Could you check a few things on this model? Use its own coordinates, in mm. A direction names the side the tool comes from. Give positions to 0.01 mm unless a question says otherwise; leave off trailing zeros. Loops run counter-clockwise (first coordinate to the right, second up) from the corner with the lowest first, then second, coordinate; pieces in that order, holes last. Notation, with made-up numbers: (66.25, 67.5) -> (80.25, 67.5) arc R21 cw to (80.25, 88.5) -> close; hole circle Ø7 at (21.25, 58.5). An arc over 180 degrees is marked (long way). Write item = value, one per line. Start each with the question number.
1) I'm going to push flat-ended pins straight in: pin 1 Ø3 at (x, z) = (4, 94.5) entering from +Y; pin 2 Ø7.5 at (x, z) = (12, -6.5) entering from +Y; pin 3 Ø5 at (x, z) = (26.5, -4.5) entering from -Y; pin 4 Ø3 at (x, z) = (26.1, 105.5) entering from -Y. Where does each tip first touch, or does it pass through?
2) I want a section at C-C (x = 6.5). List the corners of the cut face in (y, z) for me, and give its area (3 significant figures).
3) I want a section at B-B (z = 84.5). List the corners of the cut face in (x, y) for me.
4) If we mould it in two halves opening along Z, with no side actions, what happens to faces 1 (the face through (24, 13, 50)), 2 (the face through (11, 5, -9.5)), 3 (the face through (27.484, 1.528, 102.838))? For each: +Z half, -Z half, draft (parallel to the pull), parting line (faces both ways), or undercut.
5) I want a section at A-A (y = 1.5). List the corners of the cut face in (x, z) for me, and give its area (3 significant figures).
6) On a 3-axis mill with a long thin cutter (end or side, diameter ignored), from which of +Z, -Z, +X, -X, +Y, -Y can I reach the whole of each face in a straight line? I mean faces 4 (the face through (1.55, 9, -5)), 5 (the face through (21.6, 8, 50)), 6 (the face through (-5.15, 1.53, 102.57)). Say none if no direction works.
7) I need wall thicknesses on probe 1 along Z at (x, y) = (26.1, 5.5); probe 2 along Z at (x, y) = (26, 2); probe 3 along X at (y, z) = (8.25, -4.5). Which ranges of each line are inside material? Lowest first, please. Write a range as from..to.
Autodesk Fusion 360 part; units mm, degrees
sketch "Sketch1" plane through (0, 0, 0) normal (0, 1, 0) x (1, 0, 0)
  line L0 (0, 0) -> (21.6, 0)
  line L1 (21.6, 0) -> (21.6, -101)
  line L2 (21.6, -101) -> (0, -101)
  line L3 (0, -101) -> (0, 0)
  line L4 (-9.5, 9.5) -> (31.1, 9.5)
  line L5 (31.1, 9.5) -> (31.1, -110.5)
  line L6 (31.1, -110.5) -> (-9.5, -110.5)
  line L7 (-9.5, -110.5) -> (-9.5, 9.5)
  circle A0 centre (-4.5, -105.5) radius 1.7
  circle A1 centre (26.1, -105.5) radius 1.7
  circle A2 centre (26.1, 4.5) radius 1.7
  circle A3 centre (-4.5, 4.5) radius 1.7
  circle A4 centre (-4.5, 4.5) radius 3
  circle A5 centre (26.1, 4.5) radius 3
  circle A6 centre (26.1, -105.5) radius 3
  circle A7 centre (-4.5, -105.5) radius 3
  dimension "d1" = 21.6
  dimension "d2" = 101
  dimension "d3" = 40.6
  dimension "d4" = 120
  dimension "d5" = 9.5
  dimension "d6" = 9.5
  dimension "d7" = 3.4
  dimension "d8" = 3.4
  dimension "d9" = 3.4
  dimension "d10" = 3.4
  dimension "d11" = 5
  dimension "d12" = 5
  dimension "d13" = 5
  dimension "d14" = 5
  dimension "d15" = 5
  dimension "d16" = 5
  dimension "d17" = 5
  dimension "d18" = 5
  dimension "d19" = 6
  dimension "d20" = 6
  dimension "d21" = 6
  dimension "d22" = 6
extrude "Extrude1" add sketch "Sketch1" along normal blind 9.9 from surface at 3.1 contours A4 | A5 | A6 | A7 makes body 1 at (29.0963, 9.7, -4.3505) makes body 2 at (-1.5037, 9.7, -4.3505) makes body 3 at (28.6599, 9.7, 103.9357) makes body 4 at (-7.2644, 9.7, 106.6653)
extrude "Extrude2" add sketch "Sketch1" along normal blind 13 contours L4 L5 L6 L7 bodies 1 2 3 4
extrude "Extrude3" add sketch "Sketch1" along normal blind 3 contours L0 L1 L2 L3 bodies 1
sketch "Sketch2" plane through (0, 13, 0) normal (0, 1, 0) x (-1, 0, 0)
  circle A0 centre (-26.1, -4.5) radius 1.7
  circle A1 centre (4.5, 105.5) radius 1.7
  line L0 (-21.6, 101) -> (0, 101)
  line L1 (0, 101) -> (0, 0)
  line L2 (0, 0) -> (-21.6, 0)
  line L3 (-21.6, 0) -> (-21.6, 101)
  line L4 (9.5, 110.5) -> (-31.1, 110.5)
  line L5 (-31.1, 110.5) -> (-31.1, -9.5)
  line L6 (-31.1, -9.5) -> (9.5, -9.5)
  line L7 (9.5, -9.5) -> (9.5, 110.5)
  circle A2 centre (4.5, -4.5) radius 1.7
  circle A3 centre (-26.1, 105.5) radius 1.7
  line L8 (-1.55, -9.5) -> (-20.05, -9.5)
  line L9 (-20.05, -9.5) -> (-20.05, 0)
  line L10 (-20.05, 0) -> (-1.55, 0)
  line L11 (-1.55, 0) -> (-1.55, -9.5)
  dimension "d30" = 11.05
  dimension "d31" = 18.5
extrude "Extrude4" cut sketch "Sketch2" against normal blind 7.5 contours L2 L6 L8 L9 L10 L11 bodies 1
fillet "Fillet1" radius 5 4 edges at (31.1, 6.5, -9.5) (-9.5, 6.5, -9.5) (-9.5, 6.5, 110.5) (31.1, 6.5, 110.5) on bodies 1
Answer list:
q1.pin_1 = 3
q1.pin_2 = 5.5
q1.pin_3 = 3.1
q1.pin_4 = through
q2.outline = (0, -9.5) -> (5.5, -9.5) -> (5.5, 0) -> (3, 0) -> (3, 101) -> (13, 101) -> (13, 110.5) -> (0, 110.5) -> close
q2.area = 479 mm^2
q3.outline = (-9.5, 0) -> (31.1, 0) -> (31.1, 13) -> (21.6, 13) -> (21.6, 3) -> (0, 3) -> (0, 13) -> (-9.5, 13) -> close
q4.face_1 = draft
q4.face_2 = -Z half
q4.face_3 = undercut
q5.outline = (-9.5, -4.5) arc R5 ccw to (-4.5, -9.5) -> (26.1, -9.5) arc R5 ccw to (31.1, -4.5) -> (31.1, 105.5) arc R5 ccw to (26.1, 110.5) -> (-4.5, 110.5) arc R5 ccw to (-9.5, 105.5) -> close; hole circle Ø6 at (-4.5, -4.5); hole circle Ø6 at (-4.5, 105.5); hole circle Ø6 at (26.1, -4.5); hole circle Ø6 at (26.1, 105.5)
q5.area = 4,740 mm^2
q6.face_4 = -Z, +Y
q6.face_5 = +Y
q6.face_6 = -Y
q7.probe_1 = -9.5..-6.2, -2.8..103.8, 107.2..110.5
q7.probe_2 = -9.5..-7.5, -1.5..102.5, 108.5..110.5
q7.probe_3 = -9.5..-6.2, -2.8..1.55, 20.05..24.4, 27.8..31.1
